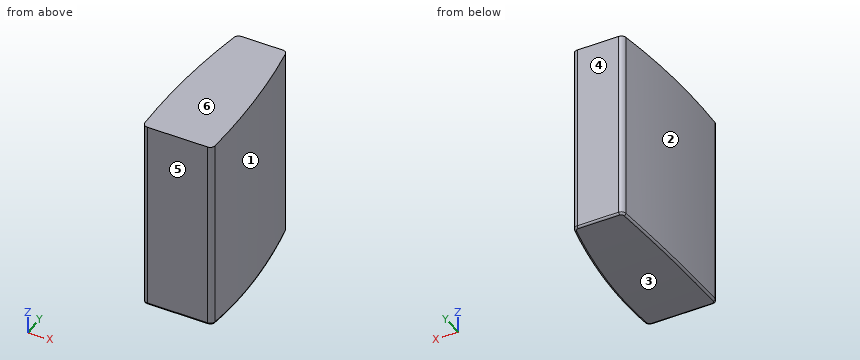
```python
from build123d import *

# Parameters (mm, degrees)
BOSS_EXTRUDE1_DEPTH = 10
CUT_EXTRUDE1_DEPTH  = 5
FILLET1_R           = 0.1


with BuildPart() as part:
    # Sketch1 → Boss-Extrude1 (new body)
    with BuildSketch(Plane.XY):
        with BuildLine():
            Line((-1.039876688, 3.9), (1.039876688, 3.9))
            ThreePointArc((1.039876688, 3.9), (1.201018652, 3.841136777), (1.286277933, 3.692266139))
            ThreePointArc((1.286277933, 3.692266139), (1.717480541, 0.028524691), (1.76066317, -3.660251846))
            ThreePointArc((1.76066317, -3.660251846), (1.683987639, -3.830364855), (1.510873459, -3.9))
            Line((1.510873459, -3.9), (-1.510873459, -3.9))
            ThreePointArc((-1.510873459, -3.9), (-1.683987639, -3.830364855), (-1.76066317, -3.660251846))
            ThreePointArc((-1.76066317, -3.660251846), (-1.717480541, 0.028524691), (-1.286277933, 3.692266139))
            ThreePointArc((-1.286277933, 3.692266139), (-1.201018652, 3.841136777), (-1.039876688, 3.9))
        make_face()
    extrude(amount=BOSS_EXTRUDE1_DEPTH)

    # Sketch2 → Cut-Extrude1 (cut, symmetric)
    with BuildSketch(Plane(origin=(0, 0, 0), x_dir=(0, 0, -1), z_dir=(1, 0, 0))):
        with BuildLine():
            Line((-0.2, 3.9), (0.726559292, 4.710927033))
            Line((0.726559292, 4.710927033), (3.434911983, -0.70577835))
            Line((3.434911983, -0.70577835), (0.497037877, -4.82568774))
            Line((0.497037877, -4.82568774), (-0.2, -3.9))
            ThreePointArc((-0.2, -3.9), (0, 0), (-0.2, 3.9))
        make_face()
    extrude(amount=CUT_EXTRUDE1_DEPTH, both=True, mode=Mode.SUBTRACT)

    # Fillet1
    fillet1_edges = [part.edges().sort_by_distance(p)[0] for p in [
        (0, -3.9, 0.2),
        (1.684192827, -3.830167686, 0.192883786),
        (1.717477583, 0.028570224, 1.0712e-05),
        (-1.717477583, 0.028570224, 1.0712e-05),
        (-1.684192827, -3.830167687, 0.192883786),
        (-1.201207437, 3.840977456, 0.19397685),
        (1.201207437, 3.840977456, 0.19397685),
        (0, 3.9, 0.2),
    ]]
    fillet(fillet1_edges, radius=FILLET1_R)


solid = part.part
```
Work out the finished part from the listing and answer in its coordinate system (mm). Face numbers are marked on the shaded views. A direction names the side the tool comes from. Round coordinates to 2 decimals unless told otherwise and drop trailing zeros. Loops run counter-clockwise (first coordinate to the right, second up) from the corner with the lowest first, then second, coordinate; pieces in that order, holes last.
(1) Each of these flat-tipped pins is pushed along its axis until it touches: P1, Ø1.5, axis at y = 0, z = 1, coming from the +X side; P2, Ø2, axis at y = 0, z = 8.5, coming from the -X side. Where does it stop, or does it pass through?
Computed values:
P1: stops at x = 1.76
P2: stops at x = -1.77
(2) The mould has two halves that part along Y. Classify the marked faces 4, 5 and 6: pulls with the +Y half, pulls with the -Y half, needs draft (parallel to the pull), parting line crosses it, or undercut.
Computed values:
face 4: pulls with the +Y half
face 5: pulls with the -Y half
face 6: needs draft
(3) The part is cut by section A-A, the plane z = 2.75. Give the vertices of the cut face in (x, y) (3 decimals).
Computed values:
outline: (-1.761, -3.66) arc R0.25 ccw to (-1.511, -3.9) - (1.511, -3.9) arc R0.25 ccw to (1.761, -3.66) arc R35 ccw to (1.286, 3.692) arc R0.25 ccw to (1.04, 3.9) - (-1.04, 3.9) arc R0.25 ccw to (-1.286, 3.692) arc R35 ccw to start
(4) For the marked faces 1, 2 and 3, determine the directions among +Z, -Z, +X, -X, +Y, -Y from which every point of the face is accessible in a straight line to the end or side of a thin tool.
Computed values:
face 1: +Z, -Z, +X
face 2: +Z, -Z, -X
face 3: -Z, +X, -X
(5) Find the intervals of material crossed by L1, parallel to Z at x = 0.15, y = -2.75; L2, parallel to Z at x = -0.3, y = 0.25; L3, parallel to X at y = -2, z = 5.5, in increasing order.
Computed values:
L1: z = 0.1 to 10
L2: z = 0 to 10
L3: x = -1.79 to 1.79
